Could you check a few things on this model? Use its own coordinates, in mm. A direction names the side the tool comes from. Coordinates: 2 decimals unless noted, no trailing zeros. Loops run counter-clockwise (first coordinate to the right, second up) from the corner with the lowest first, then second, coordinate; pieces in that order, holes last. Notation, with made-up numbers: (-35.75, -28.75) - (-17.75, -28.75) arc R19 cw to (-17.75, -6.75) - close; hole circle Ø2 at (20, -14). An arc over 180 degrees is marked (long way). One line per item, written item: value. Start each with the question number.
(1) If we section it at C-C on y = 7: Write out the boundary of the cut face in (x, z) (3 decimals).
(2) If we section it at D-D on z = 1.25: Write out the boundary of the cut face in (x, y) (3 decimals), then the cut area to 3 significant figures.
(3) If we mould it in two halves opening along Z, with no side actions, what happens to faces 4 (the face through (2, 28.575, 6)), 5 (the face through (2, 8, 0)), 6 (the face through (1.61, 12.2, 4.64)), 7 (the face through (2, 8, 12.7))? For each: pulls with the +Z half, pulls with the -Z half, needs draft (parallel to the pull), parting line crosses it, or undercut.
(4) If I drill on line 1 along Y through (x, z) = (1.1, 6.35) (3 decimals); line 2 along Y through (x, z) = (1.75, 8.75) (3 decimals); line 3 along X through (y, z) = (2.5, 6.75), over which ranges is the centre line in solid material (lowest first)? Write a range as from..to.
(5) If we section it at B-B on x = 10.5: Write out the boundary of the cut face in (y, z) (3 decimals).
(6) I'm going to push a flat-ended pin straight in: P1, Ø6, axis at x = 4.5, z = 2, coming from the -Y side. Where does the tip first touch, or does it pass through?
(7) If we section it at A-A on z = 6.35: Count the separate pieces of the cut face and the enclosed holes in it, then the cut area to 3 significant figures.
(8) On a 3-axis mill with a long thin cutter (end or side, diameter ignored), from which of +Z, -Z, +X, -X, +Y, -Y can I reach the whole of each face in a straight line? I mean faces 1 (the face through (6.35, 2, 6)), 2 (the face through (14.44, 3.175, 6.26)), 3 (the face through (25.4, 2, 6)). Say none if no direction works.
```python
from build123d import *

# Parameters (mm, degrees)
BOSS_EXTRUDE1_DEPTH = 12.7
SKETCH2_R           = 3.175
CUT_EXTRUDE1_DEPTH  = 4.175
SKETCH4_W           = 7.9375
SKETCH4_H           = 4.7625
CUT_EXTRUDE2_DEPTH  = 4.175


with BuildPart() as part:
    # Sketch1 → Boss-Extrude1 (new body)
    with BuildSketch(Plane.XY):
        Polygon((0, 0), (25.4, 0), (25.4, 3.175), (3.175, 3.175), (3.175, 28.575), (0, 28.575), align=None)
    extrude(amount=BOSS_EXTRUDE1_DEPTH)

    # Sketch2 → Cut-Extrude1 (cut, through all)
    with BuildSketch(Plane(origin=(3.175, 0, 0), x_dir=(0, 0, -1), z_dir=(1, 0, 0))):
        with Locations((-6.35, 22.225)):
            Circle(SKETCH2_R)
        with Locations((-6.35, 9.525)):
            Circle(SKETCH2_R)
    extrude(amount=-CUT_EXTRUDE1_DEPTH, mode=Mode.SUBTRACT)

    # Sketch4 → Cut-Extrude2 (cut, through all)
    with BuildSketch(Plane(origin=(0, 3.175, 0), x_dir=(1, 0, 0), z_dir=(0, 1, 0))):
        with Locations((10.31875, -6.34365)):
            Rectangle(SKETCH4_W, SKETCH4_H)
    extrude(amount=-CUT_EXTRUDE2_DEPTH, mode=Mode.SUBTRACT)


solid = part.part
```
Values:
1. outline: (0, 0) - (3.175, 0) - (3.175, 4.425) - (0, 4.425) - close; (0, 8.275) - (3.175, 8.275) - (3.175, 12.7) - (0, 12.7) - close
2. outline: (0, 0) - (25.4, 0) - (25.4, 3.175) - (3.175, 3.175) - (3.175, 28.575) - (0, 28.575) - close
2. area: 161 mm2
3. face 4: needs draft
3. face 5: pulls with the -Z half
3. face 6: undercut
3. face 7: pulls with the +Z half
4. line 1: y = 0..6.35, 12.7..19.05, 25.4..28.575
4. line 2: y = 0..7.446, 11.604..20.146, 24.304..28.575
4. line 3: x = 0..6.35, 14.29..25.4
5. outline: (0, 0) - (3.175, 0) - (3.175, 3.962) - (0, 3.962) - close; (0, 8.725) - (3.175, 8.725) - (3.175, 12.7) - (0, 12.7) - close
6. P1: stops at y = 0
7. separate pieces: 4
7. enclosed holes: 0
7. area: 95.8 mm2
8. face 1: +Y, -Y
8. face 2: +Z, -Z, +X, +Y
8. face 3: +Z, -Z, +X, +Y, -Y
